Build history of the part. All positions in model axes, mm. Face numbers are marked on the shaded views. Coordinates: 2 decimals unless noted, no trailing zeros. Order: outer loops, then holes, each group sorted by start corner. A loop starts at its lowest first (then second) coordinate and runs counter-clockwise, first axis right, second up. Notation, with made-up numbers: (-15.75, 55) - (32.25, 55) arc R22 ccw to (32.25, 77) - close; hole circle Ø3 at (-19.75, 47). An arc over 180 degrees is marked (long way). Return JSON: item names as keys, results as strings.
from build123d import *

# Parameters (mm, degrees)
SKETCH1_W              = 25
SKETCH1_H              = 25
SKETCH1_R              = 1.55
BOSS_EXTRUDE1_DEPTH    = 3
FILLET1_R              = 25
CUT_EXTRUDE1_OUTLINE_W = 12
CUT_EXTRUDE1_OUTLINE_H = 3
FILLET3_R              = 3
FILLET4_R              = 3


# Read off the part's stored shape, not the designer's step: Cut-Extrude1
with BuildPart() as part:
    # Sketch1 → Boss-Extrude1 (new body)
    with BuildSketch(Plane(origin=(0, 0, 0), x_dir=(1, 0, 0), z_dir=(0, 1, 0))):
        Rectangle(SKETCH1_W, SKETCH1_H)
        with Locations(Location((-9.5, 9.5, 0), (0, 0, 270))):
            Circle(SKETCH1_R, mode=Mode.SUBTRACT)
        with Locations(Location((-9.5, -9.5, 0), (0, 0, 270))):
            Circle(SKETCH1_R, mode=Mode.SUBTRACT)
    extrude(amount=-BOSS_EXTRUDE1_DEPTH)

    # Fillet1
    fillet1_edges = [part.edges().sort_by_distance(p)[0] for p in [
        (12.5, -1.5, 12.5),
    ]]
    fillet(fillet1_edges, radius=FILLET1_R - 0.0001)  # a hair under: the kernel refuses the full size

    # Cut-Extrude1 outline → Cut-Extrude1 (revolve, cut)
    with BuildSketch(Plane(origin=(12.5, 0, -12.5), x_dir=(1, 0, 0), z_dir=(0, 0, 1))):
        with Locations((6, -1.5)):
            Rectangle(CUT_EXTRUDE1_OUTLINE_W, CUT_EXTRUDE1_OUTLINE_H)
    revolve(axis=Axis((12.5, 0, -12.5), (0, 1, 0)), mode=Mode.SUBTRACT)

    # Fillet3
    fillet3_edges = [part.edges().sort_by_distance(p)[0] for p in [
        (9.620035077, -1.5, -0.850716673),
        (0.5, -1.5, -12.5),
    ]]
    fillet(fillet3_edges, radius=FILLET3_R)

    # Fillet4
    fillet4_edges = [part.edges().sort_by_distance(p)[0] for p in [
        (-12.5, -1.5, 12.5),
        (-12.5, -1.5, -12.5),
    ]]
    fillet(fillet4_edges, radius=FILLET4_R)


solid = part.part
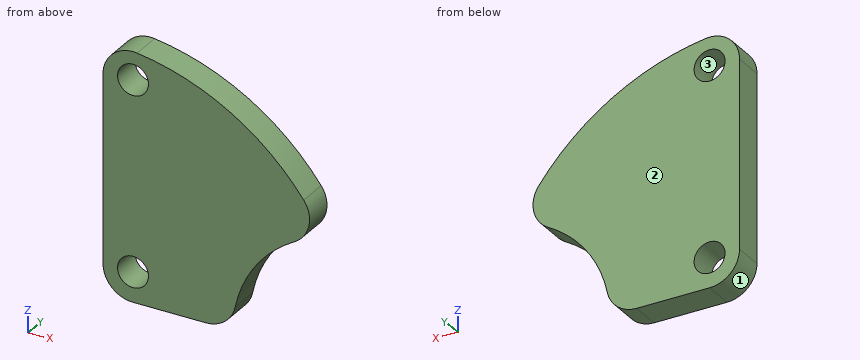
1. Cut at B-B on z = 7. Give the cut face in (x, y), plus the area to 3 significant figures.
Check values:
{"outline": "(-12.5, -3) - (3.14, -3) - (3.14, 0) - (-12.5, 0) - close", "area": "46.9 mm²"}
2. Probe L1, parallel to X at y = -1.4, z = -9.5; L2, parallel to X at y = -2.3, z = 9.5; L3, parallel to X at y = -0.7, z = -6. List the from-to ranges inside material, lowest first.
Check values:
{"L1": "-12.5 to -11.05, -7.95 to 0.88", "L2": "-12.49 to -11.05, -7.95 to -0.63", "L3": "-12.5 to 2.41"}
3. Cut at A-A on y = -1.45. State how many separate pieces and enclosed holes the cut face has, plus the area to 3 significant figures.
Check values:
{"separate pieces": "1", "enclosed holes": "2", "area": "366 mm²"}
4. Drop a flat-ended pin along its axis: pin 1 (3 mm diameter, centred on x = 1, z = 8, fed in from +Y). Give the stop position or say it passes through.
Check values:
{"pin 1": "y = 0"}
5. Mould opens along X. For the marked faces 1, 2 and 3 say: pulls with the +X half, pulls with the -X half, needs draft (parallel to the pull), parting line crosses it, or undercut.
Check values:
{"face 1": "pulls with the -X half", "face 2": "needs draft", "face 3": "undercut"}
6. Cut at C-C on x = -5. Give the cut face in (y, z), plus the area to 3 significant figures.
Check values:
{"outline": "(-3, -12.5) - (0, -12.5) - (0, 11.35) - (-3, 11.35) - close", "area": "71.5 mm²"}
